from build123d import *

# Parameters (mm, degrees)
ESQUISSE1_W        = 10
ESQUISSE1_H        = 5
BOSS_EXTRU_1_DEPTH = 5


with BuildPart() as part:
    # Esquisse1 → Boss.-Extru.1 (new body)
    with BuildSketch(Plane.XY):
        with BuildLine():
            Line((0, 22.5), (150, 22.5))
            Line((150, 22.5), (150, -22.5))
            Line((150, -22.5), (0, -22.5))
            ThreePointArc((0, -22.5), (-22.5, 0), (0, 22.5))
        make_face()
        with Locations((40, 0)):
            Rectangle(ESQUISSE1_W, ESQUISSE1_H, mode=Mode.SUBTRACT)
        with Locations((85, 0)):
            Rectangle(ESQUISSE1_W, ESQUISSE1_H, mode=Mode.SUBTRACT)
        with Locations((130, 0)):
            Rectangle(ESQUISSE1_W, ESQUISSE1_H, mode=Mode.SUBTRACT)
    extrude(amount=BOSS_EXTRU_1_DEPTH)


solid = part.part
Part model, mm, in its own coordinate system. A direction names the side the tool comes from. Give positions to 0.01 mm unless a question says otherwise; leave off trailing zeros. Loops run counter-clockwise (first coordinate to the right, second up) from the corner with the lowest first, then second, coordinate; pieces in that order, holes last. Notation, with made-up numbers: M 57.5,-5 L 91.5,-5 A21 ccw 91.5,11 Z; hole C 73.5,-37.5 d4. An arc over 180 degrees is marked long. Put each result on its own line as item: value. Start each with the question number.
1) Saw through at C-C (y = -11.5). List the corners of the cut face in (x, z).
2) Pull direction Y, two halves, no side cores. Call faces 1 (the flat face through (65, 0, 5)), 2 (the flat face through (76, -22.5, 2)), 3 (the flat face through (130, -2.5, 2)): +Y half, -Y half, draft (parallel to the pull), parting line (faces both ways), or undercut.
3) 3-axis set-ups, long thin cutter, end or side, ignore diameter. For faces 4 (the flat face through (130, 2.5, 2)), 5 (the flat face through (150, 0, 2)): which of +Z, -Z, +X, -X, +Y, -Y reach the whole face in a straight line?
4) Saw through at B-B (y = 0). List the corners of the cut face in (x, z), then the cut area to 4 significant figures.
5) Saw through at D-D (y = 18.5). List the corners of the cut face in (x, z), then the cut area to 3 significant figures.
6) Probe probe 1 along X at (y, z) = (1, 2.15); probe 2 along Y at (x, z) = (36, 1.7); probe 3 along X at (y, z) = (-16.5, 1.7). List the from-to ranges inside material, lowest first.
7) Saw through at A-A (z = 2.15). List the corners of the cut face in (x, y), then the cut area to 3 significant figures.
8) Flat gauge pins, fed straight in: pin 1 (3 mm diameter, centred on y = 10.5, z = 1.5, fed in from -X); pin 2 (1.5 mm diameter, centred on y = 1, z = 3, fed in from -X). Where does each tip first touch, or does it go through?
Numbers:
1. outline: M -19.34,0 L 150,0 L 150,5 L -19.34,5 Z
2. face 1: draft
2. face 2: -Y half
2. face 3: undercut
3. face 4: +Z, -Z
3. face 5: +Z, -Z, +X, +Y, -Y
4. outline: M -22.5,0 L 35,0 L 35,5 L -22.5,5 Z; M 45,0 L 80,0 L 80,5 L 45,5 Z; M 90,0 L 125,0 L 125,5 L 90,5 Z; M 135,0 L 150,0 L 150,5 L 135,5 Z
4. area: 712.5 mm^2
5. outline: M -12.81,0 L 150,0 L 150,5 L -12.81,5 Z
5. area: 814 mm^2
6. probe 1: -22.48 to 35, 45 to 80, 90 to 125, 135 to 150
6. probe 2: -22.5 to -2.5, 2.5 to 22.5
6. probe 3: -15.3 to 150
7. outline: M 0,-22.5 L 150,-22.5 L 150,22.5 L 0,22.5 A22.5 ccw Z; hole M 35,-2.5 L 45,-2.5 L 45,2.5 L 35,2.5 Z; hole M 80,-2.5 L 90,-2.5 L 90,2.5 L 80,2.5 Z; hole M 125,-2.5 L 135,-2.5 L 135,2.5 L 125,2.5 Z
7. area: 7,400 mm^2
8. pin 1: x = -20.62
8. pin 2: x = -22.5
